Could you check a few things on this model? Use its own coordinates, in mm. A direction names the side the tool comes from. Give positions to 0.01 mm unless a question says otherwise; leave off trailing zeros. Loops run counter-clockwise (first coordinate to the right, second up) from the corner with the lowest first, then second, coordinate; pieces in that order, holes last. Notation, with made-up numbers: M -22.75,77.25 L -15.75,77.25 A14 ccw -15.75,98.25 Z; hole C -16,16.25 d6. An arc over 180 degrees is marked long. Return JSON: item names as keys, results as strings. Group by question number.
1. If we section it at D-D (y = -364): Write out the boundary of the cut face in (x, z).
2. Please list where these lines run through material, in increasing order: line 1 (Y direction, x = 11, z = 2.95); line 2 (X direction, y = -227, z = 1.1); line 3 (X direction, y = -56, z = 0.8).
3. If we section it at A-A (x = 96.5): Write out the boundary of the cut face in (y, z).
4. If we section it at B-B (z = 3.35): Write out the boundary of the cut face in (x, y), plus the area to 3 significant figures.
5. For faces 4 (the flat face through (77.65, -317.05, 1.97)), 5 (the flat face through (82, -199, 0)), which set-ups out of +Z, -Z, +X, -X, +Y, -Y let a thin tool reach every point of the face, with its end or its side?
6. If we mould it in two halves opening along Y, with no side actions, what happens to faces 1 (the flat face through (82, -199, 4)), 2 (the flat face through (52, -130, 2)), 3 (the flat face through (69.3, -123.25, 1.97))? For each: +Y half, -Y half, draft (parallel to the pull), parting line (faces both ways), or undercut.
7. If we section it at C-C (x = 44.5): Write out the boundary of the cut face in (y, z).
Autodesk Fusion 360 part; units mm, degrees
sketch "Sketch1" plane through (0, 0, 0) normal (0, 0, 1) x (1, 0, 0)
  line L0 (0, 0) -> (20, 0)
  line L1 (20, 0) -> (120, -250)
  line L2 (120, -250) -> (70, -400)
  line L3 (70, -400) -> (50, -400)
  line L4 (4, -10) -> (14, -10)
  line L5 (53.3333, -390) -> (63.3333, -390)
  line L6 (63.3333, -386) -> (54.6667, -386)
  line L7 (100, -250) -> (54.6667, -386)
  line L8 (53.3333, -390) -> (50, -400)
  line L9 (0, 0) -> (4, -10)
  line L10 (5.6, -14) -> (100, -250)
  line L11 (14, -10) -> (14, -14)
  line L12 (5.6, -14) -> (14, -14)
  line L13 (63.3333, -390) -> (63.3333, -386)
  dimension "d4" = 400
  dimension "d5" = 50
  dimension "d6" = 50
  dimension "d7" = 250
  dimension "d9" = 20
  dimension "d10" = 20
  dimension "d11" = 20
  dimension "d12" = 10
  dimension "d13" = 4
  dimension "d14" = 10
  dimension "d15" = 10
  dimension "d16" = 4
  dimension "d17" = 10
  dimension "d27" = 4
extrude "Extrude1" add sketch "Sketch1" along normal blind 4
sketch "Sketch1 (2)" plane through (0, 0, 0) normal (0, 0, 1) x (1, 0, 0) in component "Lampi1"
component "Lampi1" placed x (1, 0, 0) y (0, 1, 0) z (0, 0, 1) at (0, 0, 0)
equation "d4 = haed_skerms"
equation "d5 = umfram_radius"
equation "d6 = umfram_radius"
equation "d7 = haed_u"
equation "d9 = Linear Dimension-6"
equation "d10 = Linear Dimension-7"
equation "d11 = Linear Dimension-8"
equation "d12 = dypt_pressfit"
equation "d13 = Linear Dimension-10"
equation "d14 = dypt_pressfit"
equation "d15 = dypt_pressfit"
equation "d16 = Linear Dimension-13"
equation "d17 = dypt_pressfit"
equation "haed_skerms = 400 mm"
equation "haed_u = 250 mm"
equation "head_l = 150 mm"
equation "dypt_pressfit = 10 mm"
equation "umfram_radius = 50 mm"
Answer:
{
 "1": {"outline": "M 62,0 L 82,0 L 82,4 L 62,4 Z"},
 "2": {"line 1": "y = -27.5 to -14, -10 to 0", "line 2": "x = 90.8 to 110.8", "line 3": "x = 22.4 to 42.4"},
 "3": {"outline": "M -320.5,0 L -260.5,0 L -260.5,4 L -320.5,4 Z; M -241.25,0 L -191.25,0 L -191.25,4 L -241.25,4 Z"},
 "4": {"outline": "M 0,0 L 4,-10 L 14,-10 L 14,-14 L 5.6,-14 L 100,-250 L 54.67,-386 L 63.33,-386 L 63.33,-390 L 53.33,-390 L 50,-400 L 70,-400 L 120,-250 L 20,0 Z", "area": "7,930 mm²"},
 "5": {"face 4": "+Z, -Z, -X", "face 5": "-Z, +X, -X, +Y, -Y"},
 "6": {"face 1": "draft", "face 2": "undercut", "face 3": "+Y half"},
 "7": {"outline": "M -111.25,0 L -61.25,0 L -61.25,4 L -111.25,4 Z"}
}
